Autodesk Inventor part; units mm, degrees
ref_plane "YZ Plane" through (0, 0, 0) normal (1, 0, 0) x (0, 1, 0)
ref_plane "XZ Plane" through (0, 0, 0) normal (0, 1, 0) x (-1, 0, 0)
ref_plane "XY Plane" through (0, 0, 0) normal (0, 0, 1) x (1, 0, 0)
sketch "Sketch1" plane through (0, 0, 0) normal (0, 1, 0) x (-1, 0, 0)
  circle A0 centre (0, 0) radius 12.7
  circle A1 centre (0, 0) radius 31.75
  dimension "d0" = 25.4
  dimension "d1" = 63.5
extrude "Extrusion1" add sketch "Sketch1" along normal blind 25.4
sketch "Sketch2" plane through (0, 25.4, 0) normal (0, 1, 0) x (1, 0, 0)
  circle A0 centre (0, 0) radius 31.75
  line L0 (-31.75, 0) -> (-26.67, 0)
  line L1 (-26.67, 0) -> (-16.51, 0)
  line L2 (-16.51, 5.08) -> (-26.67, 0)
  line L3 (-16.51, -5.08) -> (-26.67, 0)
  arc A1 (-16.51, 5.08) -> (-26.67, 0) centre (-17.3323, -5.9755) ccw
  line L4 (-26.67, 0) -> (-25.783, -10.1212)
  arc A2 (-26.67, 0) -> (-25.783, -10.1212) centre (-19.661, -4.4852) ccw
  arc A3 (-16.51, 5.08) -> (-16.51, -5.08) centre (-4.0157, 0) ccw
  arc A4 (-16.51, -5.08) -> (-25.783, -10.1212) centre (-20.2123, -9.3191) ccw
  dimension "d4" = 5.08
  dimension "d6" = 5.08
  dimension "d7" = 10.16
  dimension "d13" = 10.16
extrude "Extrusion2" cut sketch "Sketch2" against normal blind 25.4 contours A1 L2 | L2 A3 L1 | L1 A3 A4 L3 | L3 A4 L4 | L4 A4 A2 | A4 L3 | L4 A4
pattern_circular "Circular Pattern1" count 8 over 360 about axis through (0, 0, 0) along (0, 1, 0) of "Extrusion2"
properties part number "whee"
The model under review builds one solid part; all positions refer to its coordinate system, in mm. A direction names the side the tool comes from. Coordinates: 2 decimals unless noted, no trailing zeros. Loops run counter-clockwise (first coordinate to the right, second up) from the corner with the lowest first, then second, coordinate; pieces in that order, holes last. Notation, with made-up numbers: (-33, 34.25) -> (23, 34.25) arc R14 ccw to (23, 39.25) -> close; hole circle Ø5 at (55.25, 60.5). An arc over 180 degrees is marked (long way). Use a Markdown table: item, result. Add a question column.
1. To check wall thickness, follow line 1 (Z direction, x = 0, y = 16.75); line 2 (X direction, y = 21.5, z = -8); line 3 (X direction, y = 24, z = 22). State the ranges of each line that lie inside material, in increasing order.
2. Draft analysis for pull direction X (two halves, no side actions). For faces 1 (the face through (-14, 0, 0)), 2 (the face through (-3.977, 12.878, 22.215)), 3 (the face through (-12.896, 12.878, -18.521)), state which applies: pulls with the +X half, pulls with the -X half, needs draft (parallel to the pull), parting line crosses it, or undercut.
3. Add section B-B on z = -21.5. Write out the cut boundary in (x, y), plus the area to 3 significant figures.
4. Clearance check with flat-ended pins moving along their axes: pin 1 Ø3 at (x, y) = (-23.5, 12.5) entering from +Z; pin 2 Ø5 at (y, z) = (14, 20.5) entering from +X; pin 3 Ø3 at (x, y) = (7.5, 19.5) entering from -Z; pin 4 Ø8 at (y, z) = (11, 3) entering from +X. State where each tip first meets the part, or that it passes through.
5. Add section C-C on y = 17.5. Give the number of separate pieces and of enclosed holes in the cut face, plus the area to 3 significant figures.
6. Machinability: for faces 4 (the face through (-14, 25.4, 0)), 5 (the face through (-4.96, 12.88, -23.77)), which of the approach directions +Z, -Z, +X, -X, +Y, -Y give a long, thin tool a straight path to every point of the face, cutting with its end or side? Answer none if there is none.
7. Add section A-A on z = 1. Write out the cut boundary in (x, y).
Returned:
| question | item | result |
|---|---|---|
| 1 | line 1 | z = -31.75 to -26.67, -17.5 to -12.7, 12.7 to 17.5, 26.67 to 31.75 |
| 1 | line 2 | x = -30.73 to -9.86, 9.86 to 25.68, 27.2 to 30.73 |
| 1 | line 3 | x = -22.89 to -17.44, -13.22 to -4.08, 3.98 to 22.89 |
| 2 | face 1 | needs draft |
| 2 | face 2 | undercut |
| 2 | face 3 | undercut |
| 3 | outline | (-23.36, 0) -> (-3.84, 0) -> (-3.84, 25.4) -> (-23.36, 25.4) -> close; (4.3, 0) -> (13.3, 0) -> (13.3, 25.4) -> (4.3, 25.4) -> close; (17.78, 0) -> (23.36, 0) -> (23.36, 25.4) -> (17.78, 25.4) -> close |
| 3 | area | 866 mm² |
| 4 | pin 1 | stops at z = 22.89 |
| 4 | pin 2 | stops at x = 26.15 |
| 4 | pin 3 | stops at z = -31.18 |
| 4 | pin 4 | stops at x = 31.75 |
| 5 | separate pieces | 1 |
| 5 | enclosed holes | 9 |
| 5 | area | 1,940 mm² |
| 6 | face 4 | +Z, -Z, +X, -X, +Y |
| 6 | face 5 | +Y, -Y |
| 7 | outline | (-31.73, 0) -> (-27.22, 0) -> (-27.22, 25.4) -> (-31.73, 25.4) -> close; (-17.47, 0) -> (-12.66, 0) -> (-12.66, 25.4) -> (-17.47, 25.4) -> close; (12.66, 0) -> (17.47, 0) -> (17.47, 25.4) -> (12.66, 25.4) -> close; (25.95, 0) -> (31.73, 0) -> (31.73, 25.4) -> (25.95, 25.4) -> close |
